Autodesk Inventor part; units mm, degrees
ref_plane "YZ Plane" through (0, 0, 0) normal (1, 0, 0) x (0, 1, 0)
ref_plane "XZ Plane" through (0, 0, 0) normal (0, 1, 0) x (-1, 0, 0)
ref_plane "XY Plane" through (0, 0, 0) normal (0, 0, 1) x (1, 0, 0)
sketch "Sketch1" plane through (0, 0, 0) normal (0, 1, 0) x (-1, 0, 0)
  circle A0 centre (0, 0) radius 12.5
  dimension "d0" = 25
extrude "Extrusion1" add sketch "Sketch1" along normal blind 58.8
hole "ReliefTop" at (0, 58.8, 0) direction (0, -1, 0) diameter 13.97 depth 0.254 countersink diameter 14.478 countersink angle 90
hole "ReliefBottom" at (0, 0, 0) direction (0, 1, 0) diameter 13.97 depth 0.254 countersink diameter 14.478 countersink angle 90
hole "MountBottomM6" at (0, 0.254, 0) direction (0, 1, 0) diameter 4.917 depth 7.366 tip angle 118 countersink diameter 5.508 countersink angle 90
hole "MountTopM4" at (0, 58.546, 0) direction (0, -1, 0) diameter 3.242 depth 14.478 tip angle 118 countersink diameter 3.808 countersink angle 90
sketch "Sketch2" plane through (0, 0, 0) normal (0, 0, 1) x (1, 0, 0)
  circle A0 centre (0, 20) radius 3
  line L0 (-12.5, 0) -> (12.5, 0)
  line L1 (0, -4.6) -> (0, 27.6)
  point P0 (0, 0)
  dimension "d49" = 6
  dimension "d50" = 20
extrude "Extrusion2" cut sketch "Sketch2" along normal through all both and the other way through all
chamfer "Chamfer1" distance 0.313 angle 45 2 edges at (-3, 19.9998, 12.1347) (-3, 19.9998, -12.1347)
equation "\"d1\" = height"
equation "\"d5\" = reliefMinor"
equation "\"d7\" = reliefMajor"
equation "\"d10\" = reliefDepth"
equation "\"d14\" = reliefMinor"
equation "\"d16\" = reliefMajor"
equation "\"d19\" = reliefDepth"
equation "\"d25\" = chamferM6"
equation "\"d28\" = depthM6"
equation "\"d40\" = chamferM4"
equation "\"d43\" = depthM4"
equation "\"reliefDepth\" = 0.254"
equation "\"reliefMinor\" = 13.97"
equation "\"reliefMajor\" = 14.478"
equation "\"chamferM6\" = 5.508"
equation "\"chamferM4\" = 3.808"
equation "\"depthM6\" = 7.366"
equation "\"depthM4\" = 14.478"
equation "\"height\" = 58.8"
properties part number "PLS-P642H0588A00_M" material "Stainless Steel"
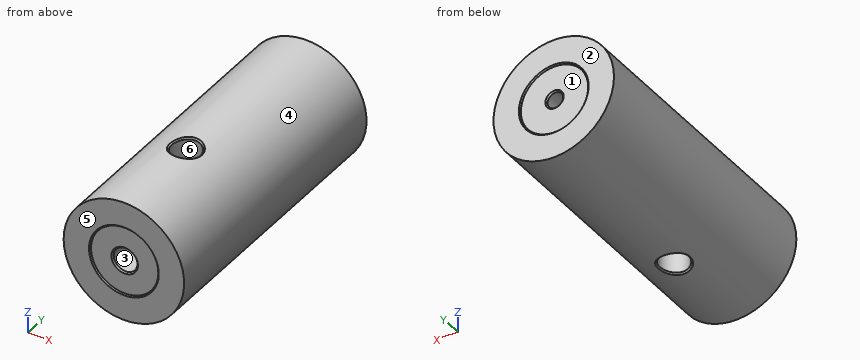
Verification items for the finished model (mm, model axes). Face numbers are marked on the shaded views. A direction names the side the tool comes from. Coordinates: 2 decimals unless noted, no trailing zeros. Order: outer loops, then holes, each group sorted by start corner. A loop starts at its lowest first (then second) coordinate and runs counter-clockwise, first axis right, second up. Notation, with made-up numbers: M 20.5,26 L 34.5,26 A31 ccw 34.5,61 Z; hole C -4.5,-11.5 d9. An arc over 180 degrees is marked long. One line per item, written item: value. Start each with the question number.
Item 1: Sectioned sample at A-A on z = -10. Record the cut outline in (x, y), then the cut area to 3 significant figures.
Item 2: Sectioned sample at D-D on x = -8. Record the cut outline in (y, z).
Item 3: Sectioned sample at C-C on y = 25. Record the cut outline in (x, z).
Item 4: Thickness scan on probe 1 along Z at (x, y) = (0, 47.5); probe 2 along Y at (x, z) = (0, -6). Record the ranges inside material, lowest first.
Item 5: Depth check by flat-ended pin: P1, Ø3.5, axis at x = 0, z = 0, coming from the +Y side; P2, Ø5, axis at x = 3, z = -1, coming from the -Y side; P3, Ø4, axis at y = 30.5, z = 9, coming from the -X side. Enter the tip coordinate at first touch or a pass-through.
Item 6: Sectioned sample at B-B on y = 52. Record the cut outline in (x, z).
Item 7: Mould release check, pull along X, two halves, no side actions. Record for the marked faces 4, 5 and 6: pulls with the +X half, pulls with the -X half, needs draft (parallel to the pull), parting line crosses it, or undercut.
Item 8: Access from +Z, -Z, +X, -X, +Y, -Y to the whole of each face (thin tool, end or side, straight path). Record for the marked faces 1, 2 and 3.
Calculated:
1. outline: M -7.5,0 L 7.5,0 L 7.5,58.8 L -7.5,58.8 Z; hole C 0,20 d6
1. area: 854 mm^2
2. outline: M 0,-9.6 L 58.8,-9.6 L 58.8,9.6 L 0,9.6 Z
3. outline: C 0,0 d25
4. probe 1: -12.5 to -1.62, 1.62 to 12.5
4. probe 2: 0.25 to 17, 23 to 58.55
5. P1: y = 58.39
5. P2: y = 0.25
5. P3: x = -10.36
6. outline: C 0,0 d25; hole C 0,0 d3.24
7. face 4: parting line crosses it
7. face 5: needs draft
7. face 6: undercut
8. face 1: +Y
8. face 2: +Z, -Z, +X, -X, +Y
8. face 3: -Y
